Autodesk Inventor part; units mm, degrees
ref_plane "YZ Plane" through (0, 0, 0) normal (1, 0, 0) x (0, 1, 0)
ref_plane "XZ Plane" through (0, 0, 0) normal (0, 1, 0) x (-1, 0, 0)
ref_plane "XY Plane" through (0, 0, 0) normal (0, 0, 1) x (1, 0, 0)
sketch "Sketch1" plane through (0, 0, 0) normal (1, 0, 0) x (0, 1, 0)
  line L0 (50.8, 28.575) -> (-50.8, 28.575)
  line L1 (-50.8, 28.575) -> (-50.8, -28.575)
  line L2 (-50.8, -28.575) -> (50.8, -28.575)
  line L3 (50.8, -28.575) -> (50.8, 28.575)
  line L4 (50.8, 28.575) -> (-50.8, -28.575) construction
  line L5 (-50.8, 28.575) -> (50.8, -28.575) construction
  point P0 (0, 0)
  dimension "d0" = 101.6
  dimension "d1" = 57.15
extrude "Extrusion1" add sketch "Sketch1" along normal blind 3.175
sketch "Sketch2" plane through (0, 0, 0) normal (-1, 0, 0) x (0, 0, 1)
  point P0 (19.8437, 30.9563)
  point P1 (19.8437, 24.6063)
  point P2 (19.8437, 18.2563)
  point P3 (19.8437, 11.9063)
  point P4 (19.8437, -13.4937)
  point P5 (19.8437, -19.8437)
  point P6 (19.8437, -26.1937)
  point P7 (19.8437, -32.5437)
  point P8 (-19.8438, -32.5437)
  point P9 (-19.8438, -26.1937)
  point P10 (-19.8438, -19.8437)
  point P11 (-19.8438, -13.4937)
  point P12 (-19.8438, 11.9063)
  point P13 (-19.8438, 18.2563)
  point P14 (-19.8438, 24.6063)
  point P15 (-19.8438, 30.9563)
hole "Hole1" at (0, 30.9563, 19.8437) at (0, 24.6063, 19.8437) at (0, 18.2563, 19.8437) at (0, 11.9063, 19.8437) at (0, -13.4937, 19.8437) at (0, -19.8437, 19.8437) at (0, -26.1937, 19.8437) at (0, -32.5437, 19.8437) at (0, -32.5437, -19.8438) at (0, -26.1937, -19.8438) at (0, -19.8437, -19.8438) at (0, -13.4937, -19.8438) at (0, 11.9063, -19.8438) at (0, 18.2563, -19.8438) at (0, 24.6063, -19.8438) at (0, 30.9563, -19.8438) direction (1, 0, 0) diameter 3.2639 end through all countersink diameter 5.715 countersink angle 82
properties part number "Ramp" material "Aluminum 6061"
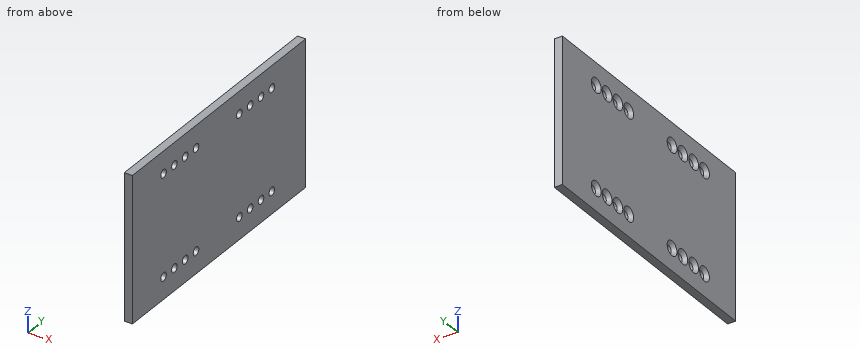
Could you check a few things on this model? Use its own coordinates, in mm. Coordinates: 2 decimals unless noted, no trailing zeros. One line per item, written item: value. Start each with the question number.
1) Imagine slicing it at A-A on x = 0.55. Count the separate pieces of the cut face and the enclosed holes in it, plus the area to 3 significant figures.
2) I'm going to push flat-ended pins straight in: pin 1 (3 mm diameter, centred on y = -26.19, z = 19.84, fed in from +X); pin 2 (4 mm diameter, centred on y = -13.49, z = 19.84, fed in from -X); pin 3 (5 mm diameter, centred on y = -19.84, z = 19.84, fed in from -X). Where does each tip first touch, or does it pass through?
3) If I drill on L1, parallel to Z at x = 1.7, y = -31.5 (3 decimals); L2, parallel to Z at x = 1, y = -18.5 (3 decimals); L3, parallel to X at y = -20, z = -17 (3 decimals), over which ranges is the centre line in solid material (lowest first)? Write a range as [from, to].
Answer list:
1. separate pieces: 1
1. enclosed holes: 16
1. area: 5,520 mm2
2. pin 1: passes through
2. pin 2: stops at x = 0.98
2. pin 3: stops at x = 0.41
3. L1: z = [-28.575, -21.098], [-18.589, 18.589], [21.098, 28.575]
3. L2: z = [-28.575, -21.309], [-18.378, 18.378], [21.309, 28.575]
3. L3: x = [0.011, 3.175]
